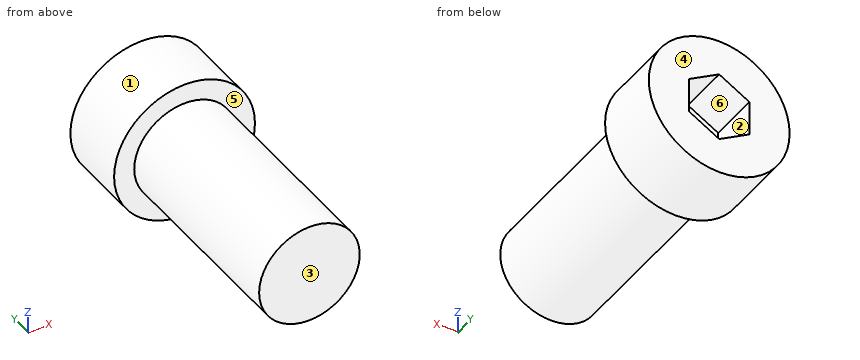
Autodesk Inventor part; units mm, degrees
ref_plane "YZ Plane" through (0, 0, 0) normal (1, 0, 0) x (0, 1, 0)
ref_plane "XZ Plane" through (0, 0, 0) normal (0, 1, 0) x (-1, 0, 0)
ref_plane "XY Plane" through (0, 0, 0) normal (0, 0, 1) x (1, 0, 0)
sketch "Sketch1" plane through (0, 0, 0) normal (0, 1, 0) x (-1, 0, 0)
  circle A0 centre (0, 0) radius 3.5
  circle A1 centre (0, 0) radius 2.5
  dimension "d0" = 7
  dimension "d1" = 5
extrude "Extrusion1" add sketch "Sketch1" against normal blind 10 contours A1
extrude "Extrusion2" add sketch "Sketch1" along normal blind 3.5 contours A0 | A1
sketch "Sketch2" plane through (0, 3.5, 0) normal (0, 1, 0) x (1, 0, 0)
  circle A0 centre (0, 0) radius 2.5
  line L0 (-1.5, -0.866) -> (-1.5, 0.866)
  line L1 (-1.5, 0.866) -> (0, 1.7321)
  line L2 (0, 1.7321) -> (1.5, 0.866)
  line L3 (1.5, 0.866) -> (1.5, -0.866)
  line L4 (1.5, -0.866) -> (0, -1.7321)
  line L5 (0, -1.7321) -> (-1.5, -0.866)
  dimension "d6" = 3
extrude "Extrusion3" cut sketch "Sketch2" against normal blind 2.5 contours L0 L1 L2 L3 L4 L5
equation "\"d0\" = D_"
equation "\"d1\" = M_"
equation "\"d2\" = L_"
equation "\"d4\" = K_"
equation "\"d6\" = S_"
equation "\"d7\" = t_"
equation "\"K_\" = 3.5"
equation "\"D_\" = 7"
equation "\"S_\" = 3"
equation "\"t_\" = 2.5"
equation "\"M_\" = 5"
equation "\"L_\" = 10"
properties part number "M5 x 10" material "Stainless Steel"
The model under review builds one solid part; all positions refer to its coordinate system, in mm. Face numbers are marked on the shaded views. A direction names the side the tool comes from. Give positions to 0.01 mm unless a question says otherwise; leave off trailing zeros. Write each loop counter-clockwise with the first axis right and the second up, starting at its lowest first coordinate (ties: lowest second). Pieces come first, ordered by that corner, then holes.
(1) For P1, Ø3, axis at x = 2.5, y = -3, coming from the +Z side; P2, Ø1.5, axis at y = -1, z = -1.5, coming from the -X side; P3, Ø3, axis at x = 1.5, y = -8.5, coming from the -Z side, all flat-tipped, find the tip position at first contact; note any pin that passes through.
(2) Consider section A-A, the plane y = 1.5. Give the boundary of the cut face in (x, z), and give its area (3 significant figures).
(3) Consider section C-C, the plane x = -2.25. Give the boundary of the cut face in (y, z).
(4) The part is to be moulded in two halves that separate along Z. For the marked faces 1, 2 and 3, say which applies: released by +Z, released by -Z, zero draft, split by the parting line, or undercut.
(5) To check wall thickness, follow L1, parallel to Y at x = -0.25, z = -0.5; L2, parallel to X at y = 2, z = -1.25; L3, parallel to Y at x = 1.5, z = 2.5. State the ranges of each line that lie inside material, in increasing order.
(6) Consider section D-D, the plane y = -2.25. Give the boundary of the cut face in (x, z).
(7) Tool access review of the marked faces 4, 5 and 6: name each direction out of +Z, -Z, +X, -X, +Y, -Y from which nothing blocks a thin tool from reaching the whole face with its end or side.
(8) Consider section B-B, the plane z = 0. Give the boundary of the cut face in (x, y).
Returned:
1. P1: stops at z = 2.29
1. P2: stops at x = -2.38
1. P3: stops at z = -2.5
2. outline: circle Ø7 at (0, 0); hole (-1.5, -0.87) - (0, -1.73) - (1.5, -0.87) - (1.5, 0.87) - (0, 1.73) - (-1.5, 0.87) - close
2. area: 30.7 mm2
3. outline: (-10, -1.09) - (0, -1.09) - (0, -2.68) - (3.5, -2.68) - (3.5, 2.68) - (0, 2.68) - (0, 1.09) - (-10, 1.09) - close
4. face 1: split by the parting line
4. face 2: undercut
4. face 3: zero draft
5. L1: y = -10 to 1
5. L2: x = -3.27 to -0.83, 0.83 to 3.27
5. L3: y = 0 to 3.5
6. outline: circle Ø5 at (0, 0)
7. face 4: +Z, -Z, +X, -X, +Y
7. face 5: -Y
7. face 6: +Y
8. outline: (-3.5, 0) - (-2.5, 0) - (-2.5, -10) - (2.5, -10) - (2.5, 0) - (3.5, 0) - (3.5, 3.5) - (1.5, 3.5) - (1.5, 1) - (-1.5, 1) - (-1.5, 3.5) - (-3.5, 3.5) - close
